Study the drawing (mm; zero at the part's minimum x, y, z) and answer. Coordinates: 2 decimals unless noted, no trailing zeros. Order: outer loops, then holes, each group sorted by start corner. A loop starts at its lowest first (then second) coordinate and runs counter-clockwise, first axis right, second up.
1. The part is cut by section A-A, the plane z = 7. Give the vertices of the cut face in (x, y), then the cut area to 3 significant figures.
2. Find the intervals of material crossed by probe 1 along X at (y, z) = (1.5, 7); probe 2 along X at (y, z) = (0.65, 5.5) (1 decimal); probe 3 along Z at (x, y) = (24.25, 0.15) (1 decimal), in increasing order.
3. Determine the mould class of the marked faces 1 and 2 for opening direction Z: +Z half, -Z half, draft (parallel to the pull), parting line (faces both ways), or undercut.
4. The part is cut by section B-B, the plane y = 0.55. Give the vertices of the cut face in (x, z).
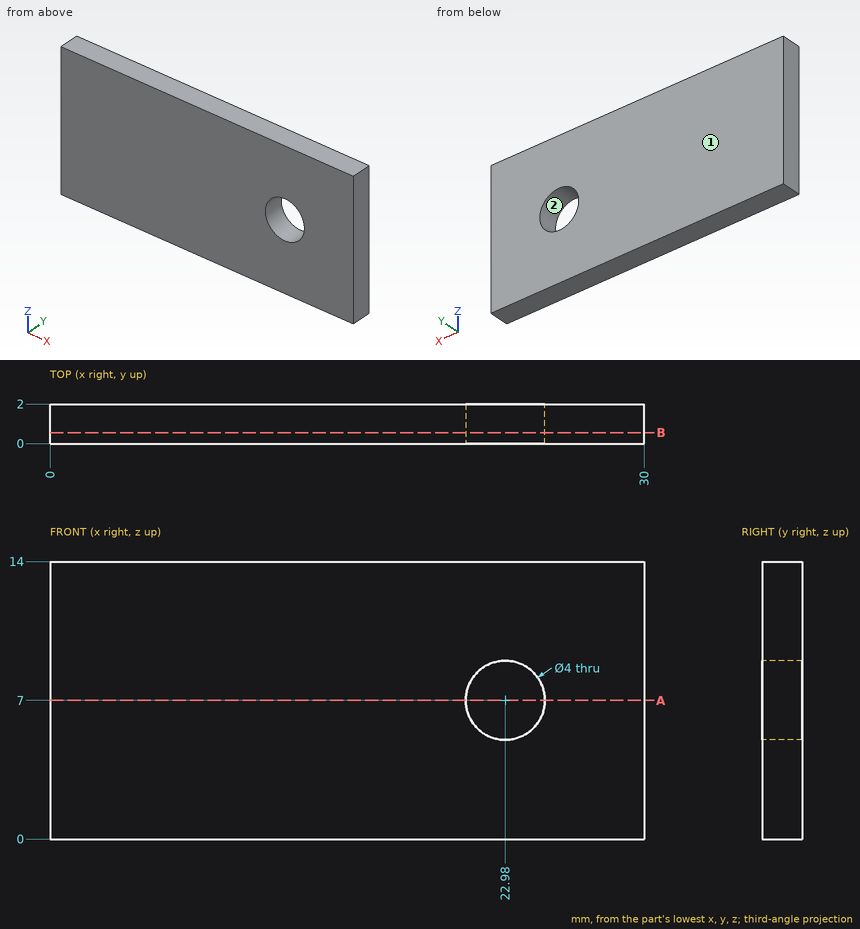
Geometry says:
1. outline: (0, 0) - (20.98, 0) - (20.98, 2) - (0, 2) - close; (24.98, 0) - (30, 0) - (30, 2) - (24.98, 2) - close
1. area: 52.0 mm2
2. probe 1: x = 0 to 20.98, 24.98 to 30
2. probe 2: x = 0 to 21.7, 24.3 to 30
2. probe 3: z = 0 to 5.5, 8.5 to 14
3. face 1: draft
3. face 2: undercut
4. outline: (0, 0) - (30, 0) - (30, 14) - (0, 14) - close; hole circle Ø4 at (22.98, 7)
